Autodesk Inventor part; units mm, degrees
ref_plane "YZ Plane" through (0, 0, 0) normal (1, 0, 0) x (0, 1, 0)
ref_plane "XZ Plane" through (0, 0, 0) normal (0, 1, 0) x (-1, 0, 0)
ref_plane "XY Plane" through (0, 0, 0) normal (0, 0, 1) x (1, 0, 0)
sketch "Sketch1" plane through (0, 0, 0) normal (0, 1, 0) x (-1, 0, 0)
  arc A0 (0.2852, 3.6388) -> (0.2852, -3.6388) centre (0, 0) ccw
  line L0 (0, 0) -> (16, 0) construction
  arc A1 (16.1875, -2.3927) -> (16.1875, 2.3927) centre (16, 0) ccw
  line L1 (0.2852, 3.6388) -> (16.1875, 2.3927)
  line L2 (0.2852, -3.6388) -> (16.1875, -2.3927)
  line L3 (5.85, 3.2028) -> (5.85, -3.2028)
  line L4 (0, 0) -> (-3.65, 0)
  circle A2 centre (0, 0) radius 1.55
  circle A3 centre (0, 0) radius 3
  circle A4 centre (0, 0) radius 5
  line L5 (0.1667, 4.9972) -> (30.1333, 3.9978)
  line L6 (0.1667, -4.9972) -> (30.1333, -3.9978)
  circle A5 centre (30, 0) radius 4
  line L7 (16, 0) -> (30, 0) construction
  circle A6 centre (30, 0) radius 1.25
  point P0 (0, 0)
  dimension "d0" = 7.3
  dimension "d1" = 4.8
  dimension "d2" = 16
  dimension "d3" = 9.5
  dimension "d4" = 3.1
  dimension "d6" = 6
  dimension "d8" = 2.5
  dimension "d18" = 10
  dimension "d19" = 8
  dimension "d20" = 30
extrude "Extrusion1" add sketch "Sketch1" against normal blind 1 contours A3 | L1 A4 L2 A0 | A0 L2 A4 L1 | A4 L5 A5 L6 L2 A1 L1 | L1 L3 L2 A4 | L1 A1 L2 L3 | A5
extrude "Extrusion2" add sketch "Sketch1" along normal blind 3 contours A0 L2 A4 L1 | A4 L5 A5 L6 L2 A1 L1 | A5 picked at (2.3095, 3.6823)
extrude "Extrusion3" add sketch "Sketch1" along normal blind 1.2 contours L1 A1 L2 L3
chamfer "Chamfer1" distance 1.2 angle 45 1 edges at (-5.85, 1.2, 0)
properties part number "Servo Arm_3DPrint"
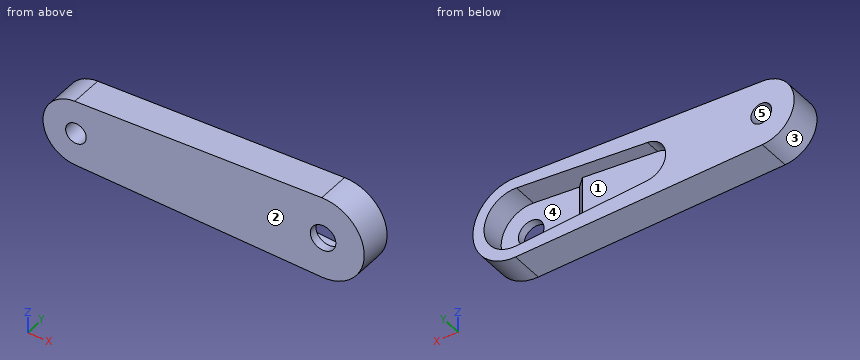
Input: part model. Units: mm. Frame: model coordinates. Face numbers are marked on the shaded views. A direction names the side the tool comes from. Give positions to 0.01 mm unless a question says otherwise; leave off trailing zeros. Order: outer loops, then holes, each group sorted by start corner. A loop starts at its lowest first (then second) coordinate and runs counter-clockwise, first axis right, second up. Notation, with made-up numbers: (-30, -19.75) - (-20, -19.75) arc R15 cw to (-20, 1.25) - close; hole circle Ø10 at (60.25, -16). An arc over 180 degrees is marked (long way). Put each result on its own line as item: value.
Item 1: Contact query for a flat-ended pin moving along its axis: pin 1 (5 mm diameter, centred on x = -14.5, z = -1.5, fed in from +Y). Output: stop coordinate, or through.
Found:
pin 1: stops at y = 3
Item 2: Access query for the marked faces 4 and 5. Directions: +Z, -Z, +X, -X, +Y, -Y. A direction counts if a zero-diameter tool reaches every point of the face in a straight line with its end or side. Return the directions, or none.
Found:
face 4: +Y
face 5: +Y, -Y
Item 3: Section query C-C, the plane y = 2.4. Return loops of the section in (x, z).
Found:
outline: (-30.13, -4) - (-0.17, -5) arc R5 ccw (long way) to (-0.17, 5) - (-30.13, 4) arc R4 ccw to start; hole circle Ø2.5 at (-30, 0); hole (-16.19, -2.39) - (-0.29, -3.64) arc R3.65 ccw (long way) to (-0.29, 3.64) - (-16.19, 2.39) arc R2.4 ccw to start
Item 4: Section query B-B, the plane y = 0.7. Return loops of the section in (x, z), then the cut area to 3 significant figures.
Found:
outline: (-30.13, -4) - (-0.17, -5) arc R5 ccw (long way) to (-0.17, 5) - (-30.13, 4) arc R4 ccw to start; hole circle Ø2.5 at (-30, 0); hole (-6.55, -3.15) - (-0.29, -3.64) arc R3.65 ccw (long way) to (-0.29, 3.64) - (-6.55, 3.15) - close
area: 264 mm^2
Item 5: Section query A-A, the plane z = 0. Count the separate pieces of the cut face and the enclosed holes in it, then the cut area to 3 significant figures.
Found:
separate pieces: 3
enclosed holes: 0
area: 91.1 mm^2
Item 6: Draft query along X for the marked faces 1, 2 and 3. Return one class per face: +X half, -X half, draft (parallel to the pull), parting line (faces both ways), or undercut.
Found:
face 1: undercut
face 2: draft
face 3: -X half
Item 7: Section query D-D, the plane x = -28. Return loops of the section in (y, z).
Found:
outline: (-1, -4.07) - (3, -4.07) - (3, 4.07) - (-1, 4.07) - close
Item 8: Ray query, L1, parallel to Z at x = -30, y = 1.9; L2, parallel to Z at x = 0, y = -0.6; L3, parallel to Y at x = -2, z = 1.25. Return the intervals inside material, ascending. Write a range as from..to.
Found:
L1: z = -4..-1.25, 1.25..4
L2: z = -5..-1.55, 1.55..5
L3: y = -1..0
